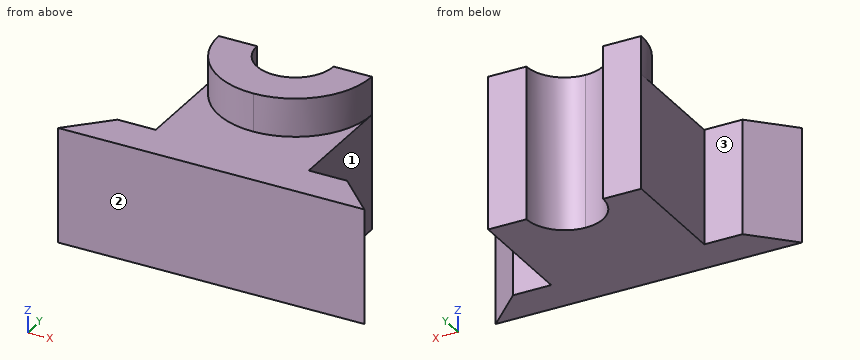
```python
from build123d import *

# Parameters (mm, degrees)
BOSS_EXTRUDE1_DEPTH = 1016
BOSS_EXTRUDE2_DEPTH = 762


with BuildPart() as part:
    # Sketch1 → Boss-Extrude1 (new body)
    with BuildSketch(Plane.XY):
        with BuildLine():
            ThreePointArc((-508, 1016), (-359.210244843, 656.789755157), (0, 508))
            Line((0, 508), (0, 762))
            ThreePointArc((0, 762), (-179.605122421, 836.394877579), (-254, 1016))
            Line((-254, 1016), (-508, 1016))
        make_face()
        with BuildLine():
            Line((0, 762), (0, 508))
            ThreePointArc((0, 508), (359.210244843, 656.789755157), (508, 1016))
            Line((508, 1016), (254, 1016))
            ThreePointArc((254, 1016), (179.605122421, 836.394877579), (0, 762))
        make_face()
    extrude(amount=BOSS_EXTRUDE1_DEPTH)

    # Sketch1_3 → Boss-Extrude2 (add)
    with BuildSketch(Plane.XY):
        with BuildLine():
            Line((-1016, 0), (0, 0))
            Line((0, 0), (0, 508))
            ThreePointArc((0, 508), (-359.210244843, 656.789755157), (-508, 1016))
            Line((-508, 1016), (-508, 254))
            Line((-508, 254), (-762, 254))
            Line((-762, 254), (-1016, 0))
        make_face()
        with BuildLine():
            Line((0, 508), (0, 0))
            Line((0, 0), (1016, 0))
            Line((1016, 0), (762, 254))
            Line((762, 254), (508, 254))
            Line((508, 254), (508, 1016))
            ThreePointArc((508, 1016), (359.210244843, 656.789755157), (0, 508))
        make_face()
    extrude(amount=BOSS_EXTRUDE2_DEPTH)


solid = part.part
```
Design review of the part built by this model. Coordinates are the model's own, in mm. Face numbers are marked on the shaded views. A direction names the side the tool comes from. Coordinates: 2 decimals unless noted, no trailing zeros. Order: outer loops, then holes, each group sorted by start corner. A loop starts at its lowest first (then second) coordinate and runs counter-clockwise, first axis right, second up. Notation, with made-up numbers: (88, -1.75) - (98, -1.75) arc R29 ccw to (98, 32.25) - close; hole circle Ø7 at (-39.75, 23). An arc over 180 degrees is marked (long way). Answer in a Markdown table with one row per item.
(1) Consider section C-C on y = 706. State the section outline as (x, z) points, plus the area to 3 significant figures.
Checked values:
| item | result |
|---|---|
| outline | (-508, 0) - (508, 0) - (508, 762) - (402.45, 762) - (402.45, 1016) - (-402.45, 1016) - (-402.45, 762) - (-508, 762) - close |
| area | 979,000 mm^2 |
(2) Clearance check with flat-ended pins moving along their axes: pin 1 (1.5 mm diameter, centred on y = 809.5, z = 298.5, fed in from -X); pin 2 (8 mm diameter, centred on y = 610.5, z = 716.5, fed in from +X); pin 3 (8 mm diameter, centred on x = -41.5, z = 393.5, fed in from +Y). State where each tip first meets the part, or that it passes through.
Checked values:
| item | result |
|---|---|
| pin 1 | x = -508 |
| pin 2 | x = 508 |
| pin 3 | y = 766.11 |
(3) For the marked faces 1, 2 and 3, list the 3-axis set-ups (+Z, -Z, +X, -X, +Y, -Y) from which the entire face can be reached by the end or side of a thin tool; tool diameter is ignored.
Checked values:
| item | result |
|---|---|
| face 1 | +Z, -Z, +X, +Y |
| face 2 | +Z, -Z, +X, -X, -Y |
| face 3 | +Z, -Z, -X, +Y |
(4) Consider section D-D on x = -645. State the section outline as (y, z) points.
Checked values:
| item | result |
|---|---|
| outline | (0, 0) - (254, 0) - (254, 762) - (0, 762) - close |
(5) Wall thickness on line 1 along X through (y, z) = (530, 384.5); line 2 along Z through (x, y) = (443.5, 512); line 3 along Y through (x, z) = (-532.5, 553): over which ranges is each line inside the solid? List them lowest first. Write a range as from..to.
Checked values:
| item | result |
|---|---|
| line 1 | -508..508 |
| line 2 | 0..762 |
| line 3 | 0..254 |
(6) Consider section A-A on y = 935.5. State the section outline as (x, z) points.
Checked values:
| item | result |
|---|---|
| outline | (-508, 0) - (-240.91, 0) - (-240.91, 1016) - (-501.58, 1016) - (-501.58, 762) - (-508, 762) - close; (240.91, 0) - (508, 0) - (508, 762) - (501.58, 762) - (501.58, 1016) - (240.91, 1016) - close |
(7) Consider section B-B on z = 369.5. State the section outline as (x, y) points, plus the area to 3 significant figures.
Checked values:
| item | result |
|---|---|
| outline | (-1016, 0) - (1016, 0) - (762, 254) - (508, 254) - (508, 1016) - (254, 1016) arc R254 cw to (-254, 1016) - (-508, 1016) - (-508, 254) - (-762, 254) - close |
| area | 1,120,000 mm^2 |
